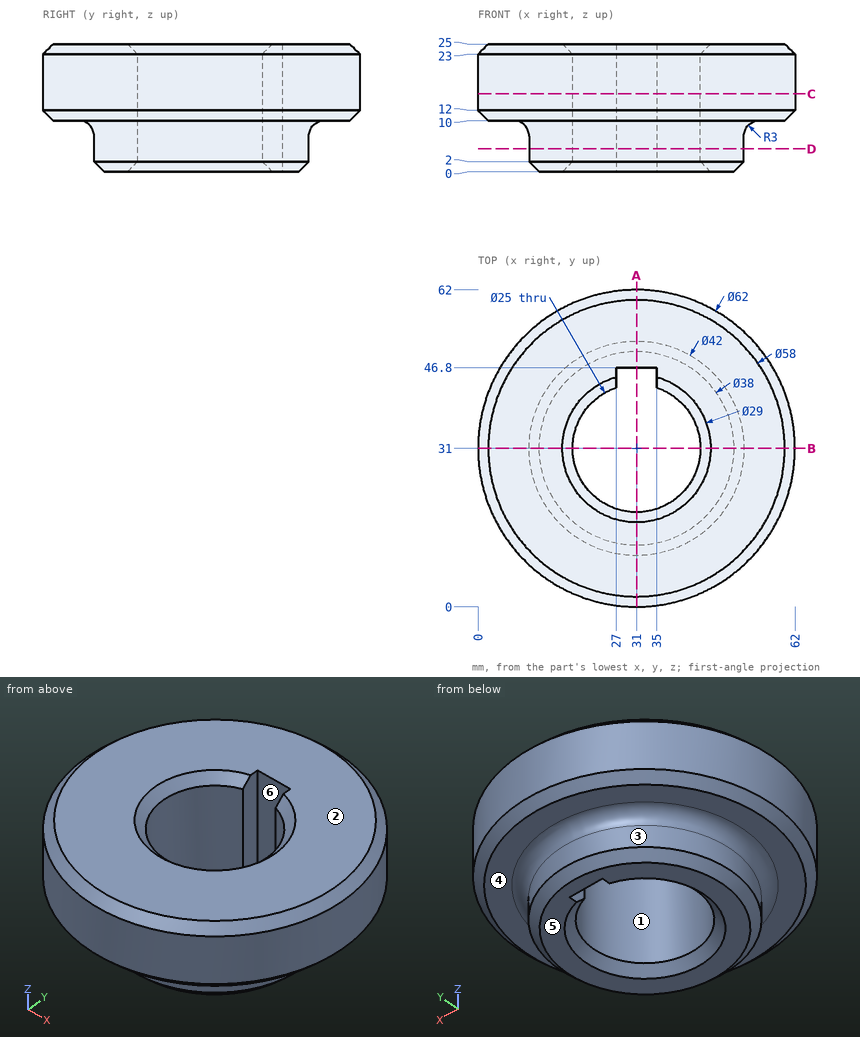
Can you work these out from the drawing? Everything is in mm from the part's minimum corner. A direction names the side the tool comes from. Round coordinates to 2 decimals unless told otherwise and drop trailing zeros. Order: outer loops, then holes, each group sorted by start corner. A loop starts at its lowest first (then second) coordinate and runs counter-clockwise, first axis right, second up. Notation, with made-up numbers: (-35, 58.25) - (18, 58.25) arc R34 ccw to (18, 90.25) - close; hole circle Ø3 at (31.25, -6.5). An arc over 180 degrees is marked (long way). Answer in a Markdown table with one row per item.
(1) Suppose I cut it at B-B, the plane y = 31. Please give me the cut outline in (x, z), plus the area to 3 significant figures.
From the geometry:
| item | result |
|---|---|
| outline | (0, 12) - (2, 10) - (7, 10) arc R3 cw to (10, 7) - (10, 2) - (12, 0) - (16.5, 0) - (18.5, 2) - (18.5, 23) - (16.5, 25) - (2, 25) - (0, 23) - close; (43.5, 2) - (45.5, 0) - (50, 0) - (52, 2) - (52, 7) arc R3 cw to (55, 10) - (60, 10) - (62, 12) - (62, 23) - (60, 25) - (45.5, 25) - (43.5, 23) - close |
| area | 709 mm2 |
(2) Suppose I cut it at C-C, the plane z = 15.25. Please give me the cut outline in (x, y).
From the geometry:
| item | result |
|---|---|
| outline | circle Ø62 at (31, 31); hole (27, 42.84) arc R12.5 ccw (long way) to (35, 42.84) - (35, 46.8) - (27, 46.8) - close |
(3) Suppose I cut it at A-A, the plane x = 31. Please give me the cut outline in (y, z).
From the geometry:
| item | result |
|---|---|
| outline | (0, 12) - (2, 10) - (7, 10) arc R3 cw to (10, 7) - (10, 2) - (12, 0) - (16.5, 0) - (18.5, 2) - (18.5, 23) - (16.5, 25) - (2, 25) - (0, 23) - close; (46.8, 0) - (50, 0) - (52, 2) - (52, 7) arc R3 cw to (55, 10) - (60, 10) - (62, 12) - (62, 23) - (60, 25) - (46.8, 25) - close |
(4) If we mould it in two halves opening along X, with no side actions, what happens to the marked faces 1, 2 and 3? For each: released by +X, released by -X, zero draft, split by the parting line, or undercut.
From the geometry:
| item | result |
|---|---|
| face 1 | undercut |
| face 2 | zero draft |
| face 3 | split by the parting line |
(5) Which directions (+Z, -Z, +X, -X, +Y, -Y) give clear straight access to the entire face, cutting with the end or side of a thin tool? Please do the marked faces 4, 5 and 6.
From the geometry:
| item | result |
|---|---|
| face 4 | -Z |
| face 5 | -Z, +X, -X, +Y, -Y |
| face 6 | +Z, -Z |
(6) Please list where these lines run through material, in increasing order: L1, parallel to Y at x = 31, z = 16.75; L2, parallel to Z at x = 57.5, y = 34.5; L3, parallel to X at y = 19.5, z = 9.5. Write a range as from..to.
From the geometry:
| item | result |
|---|---|
| L1 | y = 0..18.5, 46.8..62 |
| L2 | z = 10..25 |
| L3 | x = 11.85..26.1, 35.9..50.15 |
(7) Suppose I cut it at D-D, the plane z = 4.5. Please give me the cut outline in (x, y).
From the geometry:
| item | result |
|---|---|
| outline | circle Ø42 at (31, 31); hole (27, 42.84) arc R12.5 ccw (long way) to (35, 42.84) - (35, 46.8) - (27, 46.8) - close |
(8) For P1, Ø4, axis at y = 45, z = 3, coming from the +X side; P2, Ø4.5, axis at y = 45, z = 18, coming from the -X side; P3, Ø12, axis at x = 43.5, y = 10.5, coming from the -Z side; P4, Ø8, axis at y = 46, z = 21, coming from the -X side, each with a flat end and sliding along its axis, tell me the tip position at first contact or that it passes through.
From the geometry:
| item | result |
|---|---|
| P1 | stops at x = 48.23 |
| P2 | stops at x = 2.31 |
| P3 | stops at z = 0 |
| P4 | stops at x = 2.02 |
